Design review of the part built by this model. Coordinates are the model's own, in mm. A direction names the side the tool comes from. Round coordinates to 2 decimals unless told otherwise and drop trailing zeros. Order: outer loops, then holes, each group sorted by start corner. A loop starts at its lowest first (then second) coordinate and runs counter-clockwise, first axis right, second up.
Autodesk Inventor part; units mm, degrees
ref_plane "YZ Plane" through (0, 0, 0) normal (1, 0, 0) x (0, 1, 0)
ref_plane "XZ Plane" through (0, 0, 0) normal (0, 1, 0) x (-1, 0, 0)
ref_plane "XY Plane" through (0, 0, 0) normal (0, 0, 1) x (1, 0, 0)
sketch "Skizze1" plane through (0, 0, 0) normal (0, 1, 0) x (-1, 0, 0)
  line L0 (12.5, -9) -> (-12.5, -9)
  line L1 (-12.5, -9) -> (-12.5, 9)
  line L2 (-12.5, 9) -> (12.5, 9)
  line L3 (12.5, 9) -> (12.5, -9)
  line L4 (12.5, -9) -> (-12.5, 9) construction
  line L5 (-12.5, -9) -> (12.5, 9) construction
  line L6 (8, -5) -> (-8, -5)
  line L7 (-8, -5) -> (-8, 2.8)
  line L8 (-8, 2.8) -> (8, 2.8)
  line L9 (8, 2.8) -> (8, -5)
  line L10 (0, 2.8) -> (0, -5) construction
  point P0 (0, 0)
  point P1 (0, 0)
  dimension "d0" = 25
  dimension "d1" = 18
  dimension "d23" = 16
  dimension "d28" = 4
  dimension "d29" = 7.8
extrude "Extrusion1" add sketch "Skizze1" along normal mid plane 5
sketch "Skizze2" plane through (0, -2.5, 0) normal (0, -1, 0) x (1, 0, 0)
  line L0 (-10.5, 7) -> (10.5, 7) construction
  line L1 (10.5, 7) -> (10.5, -6.5) construction
  line L2 (10.5, -6.5) -> (-10.5, -6.5) construction
  line L3 (-10.5, -6.5) -> (-10.5, 7) construction
  line L4 (0, 12.6) -> (0, -12.6)
  line L5 (12.5, 9) -> (-12.5, 9)
  point P0 (0, 0)
  dimension "d4" = 21
  dimension "d5" = 13.5
  dimension "d6" = 2
hole "Bohrung1" at (-10.5, -2.5, 7) at (10.5, -2.5, 7) at (10.5, -2.5, -6.5) at (-10.5, -2.5, -6.5) direction (0, 1, 0) diameter 1.567 end through all
sketch "Skizze3" plane through (12.5, 2.5, -9) normal (0, 0, -1) x (-1, 0, 0)
  line L0 (25, -5) -> (25, 0)
  line L1 (0, 0) -> (25, 0)
  line L2 (0, 0) -> (0, -5)
  line L3 (25, -5) -> (0, -5)
  line L4 (25, -2.5) -> (0, -2.5) construction
  line L5 (0, -5) -> (25, -5) construction
  line L6 (12.5, -5) -> (12.5, 0) construction
  line L7 (25, 0) -> (0, 0) construction
  point P0 (12.5, -2.5)
  point P1 (18.5, -2.5)
  point P2 (6.5, -2.5)
  dimension "d14" = 12
hole "Bohrung2" at (-6, 0, -9) at (6, 0, -9) direction (0, 0, 1) diameter 2.459 depth 4
fillet "Rundung1" radius 2 2 edges at (-12.5, 0, 9) (12.5, 0, 9)
sketch "Skizze4" plane through (0, -2.5, 0) normal (0, -1, 0) x (1, 0, 0)
  line L0 (-9, 0.5) -> (9, 0.5) construction
  line L1 (-9, -1.8) -> (9, -1.8)
  line L2 (9, 2.8) -> (-9, 2.8)
  arc A0 (-9, 2.8) -> (-9, -1.8) centre (-9, 0.5) ccw
  arc A1 (9, -1.8) -> (9, 2.8) centre (9, 0.5) ccw
  line L3 (0, 12.6) -> (0, -12.6)
  line L4 (-12.5, -9) -> (12.5, -9)
  point P0 (0, 0)
  point P1 (0, 0.5)
  dimension "d24" = 4.6
  dimension "d25" = 18
  dimension "d30" = 9.5
extrude "Extrusion2" cut sketch "Skizze4" against normal blind 2
properties part number "Kamerahalter Vorne" material "PC/ABS-Kunststoff"
1) Take a section at D-D on x = -6. Give the boundary of the cut face in (y, z).
Results:
outline: (-2.5, -9) - (-1.23, -9) - (-1.23, -5) - (-2.5, -5) - close; (-2.5, 2.8) - (2.5, 2.8) - (2.5, 9) - (-2.5, 9) - close; (1.23, -9) - (2.5, -9) - (2.5, -5) - (1.23, -5) - close
2) Clearance check with flat-ended pins moving along their axes: P1, Ø1, axis at x = 9.5, z = 0, coming from the -Y side; P2, Ø1.5, axis at x = -6, y = 0, coming from the -Z side; P3, Ø1.4, axis at x = -10.5, z = 7, coming from the +Y side. State where each tip first meets the part, or that it passes through.
Results:
P1: stops at y = -0.5
P2: stops at z = 2.8
P3: passes through
3) Take a section at C-C on x = -2.75. Give the boundary of the cut face in (y, z).
Results:
outline: (-2.5, -9) - (2.5, -9) - (2.5, -5) - (-2.5, -5) - close; (-2.5, 2.8) - (2.5, 2.8) - (2.5, 9) - (-2.5, 9) - close
4) The part is to be moulded in two halves that separate along X. For faces 1 (the face through (0, 0, 9)), 2 (the face through (11.195, 0.035, -6.862)), 3 (the face through (-11.93, 0.04, 8.4)), say which applies: released by +X, released by -X, zero draft, split by the parting line, or undercut.
Results:
face 1: zero draft
face 2: undercut
face 3: released by -X
5) Take a section at B-B on y = 0. Give the boundary of the cut face in (x, z), plus the area to 3 significant figures.
Results:
outline: (-12.5, -9) - (-7.23, -9) - (-7.23, -5) - (-8, -5) - (-8, 2.8) - (8, 2.8) - (8, -5) - (7.23, -5) - (7.23, -9) - (12.5, -9) - (12.5, 7) arc R2 ccw to (10.5, 9) - (-10.5, 9) arc R2 ccw to (-12.5, 7) - close; (-4.77, -9) - (4.77, -9) - (4.77, -5) - (-4.77, -5) - close; hole circle Ø1.57 at (-10.5, -6.5); hole circle Ø1.57 at (-10.5, 7); hole circle Ø1.57 at (10.5, -6.5); hole circle Ø1.57 at (10.5, 7)
area: 296 mm2
6) For faces 4 (the face through (7.2, -0.27, -6.97)), 5 (the face through (0, 2.5, 4)), 6 (the face through (8, 1, -2)), 7 (the face through (-8.5, -1.5, -1.8)), list the 3-axis set-ups (+Z, -Z, +X, -X, +Y, -Y) from which the entire face can be reached by the end or side of a thin tool; tool diameter is ignored.
Results:
face 4: -Z
face 5: +Z, -Z, +X, -X, +Y
face 6: +Y, -Y
face 7: -Y
7) To check wall thickness, follow line 1 along Z through (x, y) = (10.5, 1.3); line 2 along Z through (x, y) = (4.25, 0.65); line 3 along X through (y, z) = (0.25, -6.5). State the ranges of each line that lie inside material, in increasing order.
Results:
line 1: z = -9 to -7.28, -5.72 to 6.22, 7.78 to 9
line 2: z = -9 to -5, 2.8 to 9
line 3: x = -12.5 to -11.28, -9.72 to -7.2, -4.8 to 4.8, 7.2 to 9.72, 11.28 to 12.5
8) Take a section at A-A on z = -6.5. Give the boundary of the cut face in (x, y).
Results:
outline: (-12.5, -2.5) - (-11.28, -2.5) - (-11.28, 2.5) - (-12.5, 2.5) - close; (-9.72, -2.5) - (9.72, -2.5) - (9.72, 2.5) - (-9.72, 2.5) - close; (11.28, -2.5) - (12.5, -2.5) - (12.5, 2.5) - (11.28, 2.5) - close; hole circle Ø2.46 at (-6, 0); hole circle Ø2.46 at (6, 0)
